Source: CAD feature listing. Evaluate the final solid. Frame: model axes, mm. A direction names the side the tool comes from. Give positions to 0.01 mm unless a question says otherwise; leave off trailing zeros. Order: outer loops, then holes, each group sorted by start corner. A loop starts at its lowest first (then second) coordinate and runs counter-clockwise, first axis right, second up. Notation, with made-up numbers: (47, 31) - (91, 31) arc R25 ccw to (91, 54) - close; hole circle Ø6 at (77.5, -27.75). An arc over 180 degrees is marked (long way). Write each question's results on one line, items separated by ' | '. Start each with the question number.
Item 1: Section B-B on y = -43. Output: boundary loops of the cut face in (x, z).
Item 2: Set-up query: faces 1 (the flat face through (140.988, -33, 15)), 2 (the flat face through (2, 5.511, 15)), 3 (the flat face through (2, -32, 5)). Return all of +Z, -Z, +X, -X, +Y, -Y with unobstructed straight access to the full face (end or side cutting, diameter ignored); none if empty.
Item 3: Section A-A on z = 19. Output: boundary loops of the cut face in (x, y), and give its area (3 significant figures).
Item 4: Contact query for flat-ended pins moving along their axis: pin 1 Ø1 at (y, z) = (1.5, 17) entering from +X; pin 2 Ø1 at (x, z) = (96, 13) entering from +Y; pin 3 Ø4 at (x, y) = (-109.5, -16) entering from +Z. Output: stop coordinate, or through.
Item 5: Mould query, pull axis Y, two halves, no side actions, for faces 4 (the flat face through (2, 0, 15)), 5 (the flat face through (2, -69.489, 15)), 6 (the flat face through (-134.012, -33, 15)). Classes: released by +Y, released by -Y, zero draft, split by the parting line, or undercut.
Item 6: Section C-C on x = 98.5. Output: boundary loops of the cut face in (y, z), and give its area (3 significant figures).
Item 7: Line query: line 1 along Y through (x, z) = (-66.5, 21.5); line 2 along X through (y, z) = (-46.5, 6); line 3 along Z through (x, y) = (134.5, -43.5). Output: solid intervals per line, ascending.
```python
from build123d import *

# Parameters (mm, degrees)
SKETCH1_W           = 285
SKETCH1_H           = 85
BOSS_EXTRUDE1_DEPTH = 5
SKETCH2_W           = 275
SKETCH2_H           = 75
BOSS_EXTRUDE2_DEPTH = 20
SKETCH3_W           = 265
SKETCH3_H           = 65
CUT_EXTRUDE1_DEPTH  = 20


with BuildPart() as part:
    # Sketch1 → Boss-Extrude1 (new body)
    with BuildSketch(Plane.XY):
        with Locations((3.487762238, -31.988636364)):
            Rectangle(SKETCH1_W, SKETCH1_H)
    extrude(amount=BOSS_EXTRUDE1_DEPTH)

    # Sketch2 → Boss-Extrude2 (add)
    with BuildSketch(Plane.XY.offset(5)):
        with Locations((3.487762238, -31.988636364)):
            Rectangle(SKETCH2_W, SKETCH2_H)
    extrude(amount=BOSS_EXTRUDE2_DEPTH)

    # Sketch3 → Cut-Extrude1 (cut)
    with BuildSketch(Plane.XY.offset(25)):
        with Locations((3.487762238, -32.5)):
            Rectangle(SKETCH3_W, SKETCH3_H)
    extrude(amount=-CUT_EXTRUDE1_DEPTH, mode=Mode.SUBTRACT)


solid = part.part
```
Evaluation:
1) outline: (-139.01, 0) - (145.99, 0) - (145.99, 5) - (140.99, 5) - (140.99, 25) - (135.99, 25) - (135.99, 5) - (-129.01, 5) - (-129.01, 25) - (-134.01, 25) - (-134.01, 5) - (-139.01, 5) - close
2) face 1: +Z, +X, +Y, -Y | face 2: +Z, +X, -X, +Y | face 3: +Z
3) outline: (-134.01, -69.49) - (140.99, -69.49) - (140.99, 5.51) - (-134.01, 5.51) - close; hole (-129.01, -65) - (135.99, -65) - (135.99, 0) - (-129.01, 0) - close | area: 3,400 mm^2
4) pin 1: stops at x = 140.99 | pin 2: stops at y = 5.51 | pin 3: stops at z = 5
5) face 4: undercut | face 5: released by -Y | face 6: zero draft
6) outline: (-74.49, 0) - (10.51, 0) - (10.51, 5) - (5.51, 5) - (5.51, 25) - (0, 25) - (0, 5) - (-65, 5) - (-65, 25) - (-69.49, 25) - (-69.49, 5) - (-74.49, 5) - close | area: 625 mm^2
7) line 1: y = -69.49 to -65, 0 to 5.51 | line 2: x = -134.01 to -129.01, 135.99 to 140.99 | line 3: z = 0 to 5
